Geometry: final body of the model. Coordinates: model frame, mm. Face numbers are marked on the shaded views. A direction names the side the tool comes from. Give positions to 0.01 mm unless a question says otherwise; leave off trailing zeros. Write each loop counter-clockwise with the first axis right and the second up, starting at its lowest first coordinate (ties: lowest second). Pieces come first, ordered by that corner, then holes. Notation, with made-up numbers: M -15,29 L -1,29 A22 cw -1,59 Z; hole C 84.5,-18.75 d10. An arc over 180 degrees is marked long. Use a Markdown table: item, result. Add a question column.
1) Section D-D on x = 4.5. Return the cut outline in (y, z), then the cut area to 3 significant figures.
2) Draft query along X for the marked faces 3, 4, 5 and 6. Return one class per face: +X half, -X half, draft (parallel to the pull), parting line (faces both ways), or undercut.
3) Set-up query: the marked faces 1 and 2. Return all of +Z, -Z, +X, -X, +Y, -Y with unobstructed straight access to the full face (end or side cutting, diameter ignored); none if empty.
4) Section B-B on z = 2.4. Return the cut outline in (x, y).
5) Pin query (flat end, axial travel): pin 1 (1.6 mm diameter, centred on y = 19, z = 1, fed in from +X); pin 2 (2 mm diameter, centred on x = 8.5, z = 1.5, fed in from -Y); pin 3 (2 mm diameter, centred on x = 15.5, z = 2, fed in from +Y). Return the tip coordinate at first contact, or that it passes through.
6) Line query: line 1 (X direction, y = 1, z = 3.3); line 2 (Y direction, x = 10, z = 0.9); line 3 (Y direction, x = 5, z = 1.55). Output: solid intervals per line, ascending.
7) Section C-C on x = 10.75. Return the cut outline in (y, z).
8) Section A-A on y = 2.5. Return the cut outline in (x, z), then the cut area to 3 significant figures.
```python
from build123d import *

# Parameters (mm, degrees)
SKETCH_2_W          = 18
SKETCH_2_H          = 21.5
EXTRUDE_1_DEPTH     = 4
SKETCH_3_W          = 12
SKETCH_3_H          = 17.5
CUT_EXTRUDE_1_DEPTH = 29.324018077
FILLET_1_R          = 5
FILLET_2_R          = 5
SKETCH_4_W          = 4
SKETCH_4_H          = 2
CUT_EXTRUDE_2_DEPTH = 29.324018077


with BuildPart() as part:
    # ｽｹｯﾁ2 → ﾎﾞｽ - 押し出し1 (new body)
    with BuildSketch(Plane.XY):
        with Locations((9, 10.75)):
            Rectangle(SKETCH_2_W, SKETCH_2_H)
    extrude(amount=EXTRUDE_1_DEPTH)

    # ｽｹｯﾁ3 → ｶｯﾄ - 押し出し1 (cut, through all)
    with BuildSketch(Plane.XY.offset(4)):
        with Locations((9, 8.75)):
            Rectangle(SKETCH_3_W, SKETCH_3_H)
    extrude(amount=-CUT_EXTRUDE_1_DEPTH, mode=Mode.SUBTRACT)

    # ﾌｨﾚｯﾄ1
    fillet_1_edges = [part.edges().sort_by_distance(p)[0] for p in [
        (3, 17.5, 2),
        (15, 17.5, 2),
    ]]
    fillet(fillet_1_edges, radius=FILLET_1_R)

    # ﾌｨﾚｯﾄ2
    fillet_2_edges = [part.edges().sort_by_distance(p)[0] for p in [
        (0, 21.5, 2),
        (18, 21.5, 2),
    ]]
    fillet(fillet_2_edges, radius=FILLET_2_R)

    # ｽｹｯﾁ4 → ｶｯﾄ - 押し出し2 (cut, through all)
    with BuildSketch(Plane.XY.offset(4)):
        with Locations((9, 19.400947982)):
            Rectangle(SKETCH_4_W, SKETCH_4_H)
    extrude(amount=-CUT_EXTRUDE_2_DEPTH, mode=Mode.SUBTRACT)


solid = part.part
```
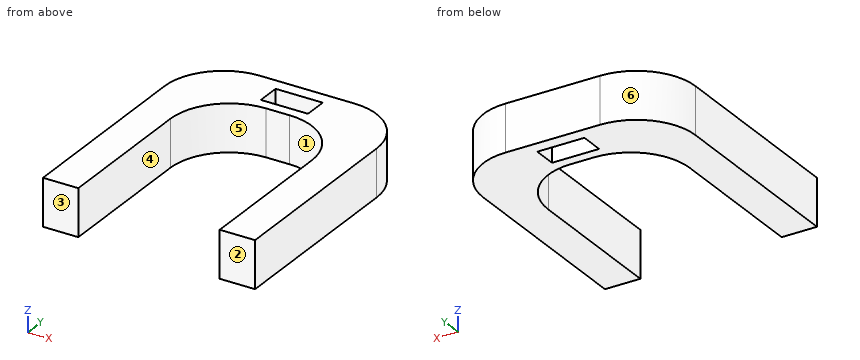
Found:
| question | item | result |
|---|---|---|
| 1 | outline | M 16.07,0 L 21.47,0 L 21.47,4 L 16.07,4 Z |
| 1 | area | 21.6 mm² |
| 2 | face 3 | draft |
| 2 | face 4 | undercut |
| 2 | face 5 | undercut |
| 2 | face 6 | -X half |
| 3 | face 1 | +Z, -Z, -Y |
| 3 | face 2 | +Z, -Z, +X, -X, -Y |
| 4 | outline | M 0,0 L 3,0 L 3,12.5 A5 cw 8,17.5 L 10,17.5 A5 cw 15,12.5 L 15,0 L 18,0 L 18,16.5 A5 ccw 13,21.5 L 5,21.5 A5 ccw 0,16.5 Z; hole M 7,18.4 L 11,18.4 L 11,20.4 L 7,20.4 Z |
| 5 | pin 1 | x = 17.7 |
| 5 | pin 2 | y = 17.47 |
| 5 | pin 3 | y = 21.27 |
| 6 | line 1 | 0 to 3, 15 to 18 |
| 6 | line 2 | 17.5 to 18.4, 20.4 to 21.5 |
| 6 | line 3 | 16.5 to 21.5 |
| 7 | outline | M 17.44,0 L 18.4,0 L 18.4,4 L 17.44,4 Z; M 20.4,0 L 21.5,0 L 21.5,4 L 20.4,4 Z |
| 8 | outline | M 0,0 L 3,0 L 3,4 L 0,4 Z; M 15,0 L 18,0 L 18,4 L 15,4 Z |
| 8 | area | 24.0 mm² |
